For this review, take the finished solid that the model builds, in its own axes (mm). A direction names the side the tool comes from. Round coordinates to 2 decimals unless told otherwise and drop trailing zeros. Order: outer loops, then holes, each group sorted by start corner. A loop starts at its lowest first (then second) coordinate and runs counter-clockwise, first axis right, second up. Notation, with made-up numbers: (-6.75, 82.5) -> (41.25, 82.5) arc R13 ccw to (41.25, 92.5) -> close; hole circle Ø6 at (-21.75, -14). An arc over 180 degrees is marked (long way). Answer in a Markdown table with one row per item.
```python
from build123d import *

# Parameters (mm, degrees)
F1_DEPTH = 3.175


with BuildPart() as f1:
    # F0 (on Top) → F1 (new body)
    with BuildSketch(Plane.XY):
        with BuildLine():
            Line((-6.35, 51.198438), (-6.35, -101.6))
            Line((-6.35, -101.6), (-1.5875, -101.6))
            Line((-1.5875, -101.6), (-1.5875, 38.1))
            Line((-1.5875, 38.1), (1.5875, 38.1))
            Line((1.5875, 38.1), (1.5875, -101.6))
            Line((1.5875, -101.6), (6.35, -101.6))
            Line((6.35, -101.6), (6.35, 51.198438))
            ThreePointArc((6.35, 51.198438), (16.414418, 53.524987), (25.800126, 57.839361))
            Line((25.800126, 57.839361), (53.881537, 47.718463))
            Line((53.881537, 47.718463), (43.760639, 75.799874))
            ThreePointArc((43.760639, 75.799874), (46.93308, 82.159682), (49.186888, 88.9))
            Line((49.186888, 88.9), (76.2, 101.6))
            Line((76.2, 101.6), (49.186888, 114.3))
            ThreePointArc((49.186888, 114.3), (46.93308, 121.040318), (43.760639, 127.400126))
            Line((43.760639, 127.400126), (53.881537, 155.481537))
            Line((53.881537, 155.481537), (25.800126, 145.360639))
            ThreePointArc((25.800126, 145.360639), (19.440318, 148.53308), (12.7, 150.786888))
            Line((12.7, 150.786888), (0, 177.8))
            Line((0, 177.8), (-12.7, 150.786888))
            ThreePointArc((-12.7, 150.786888), (-19.440318, 148.53308), (-25.800126, 145.360639))
            Line((-25.800126, 145.360639), (-53.881537, 155.481537))
            Line((-53.881537, 155.481537), (-43.760639, 127.400126))
            ThreePointArc((-43.760639, 127.400126), (-46.93308, 121.040318), (-49.186888, 114.3))
            Line((-49.186888, 114.3), (-76.2, 101.6))
            Line((-76.2, 101.6), (-49.186888, 88.9))
            ThreePointArc((-49.186888, 88.9), (-46.93308, 82.159682), (-43.760639, 75.799874))
            Line((-43.760639, 75.799874), (-53.881537, 47.718463))
            Line((-53.881537, 47.718463), (-25.800126, 57.839361))
            ThreePointArc((-25.800126, 57.839361), (-16.414418, 53.524987), (-6.35, 51.198438))
        make_face()
    extrude(amount=F1_DEPTH)


solid = f1.part
```
Q1. Tool access review of faces 1 (the face through (62.5, 95.16, 1.57)), 2 (the face through (-39.64, 150.35, 1.57)), 3 (the face through (-62.5, 108.04, 1.57)), 4 (the face through (16.28, 53.48, 1.57)): name each direction out of +Z, -Z, +X, -X, +Y, -Y from which nothing blocks a thin tool from reaching the whole face with its end or side.
Answer key:
| item | result |
|---|---|
| face 1 | +Z, -Z, +X |
| face 2 | +Z, -Z, +Y |
| face 3 | +Z, -Z, -X |
| face 4 | +Z, -Z, -Y |
Q2. Take a section at C-C, the plane y = 54. Write out the cut boundary in (x, z) (3 decimals).
Answer key:
| item | result |
|---|---|
| outline | (-51.618, 0) -> (-36.453, 0) -> (-36.453, 3.175) -> (-51.618, 3.175) -> close; (-17.745, 0) -> (17.745, 0) -> (17.745, 3.175) -> (-17.745, 3.175) -> close; (36.453, 0) -> (51.618, 0) -> (51.618, 3.175) -> (36.453, 3.175) -> close |
Q3. The part is to be moulded in two halves that separate along Y. For faces 5 (the face through (46.895, 82.068, 1.565)), 6 (the face through (-40.037, 52.708, 1.565)), 7 (the face through (19.532, 148.495, 1.565)), say which applies: +Y half, -Y half, draft (parallel to the pull), parting line (faces both ways), or undercut.
Answer key:
| item | result |
|---|---|
| face 5 | undercut |
| face 6 | -Y half |
| face 7 | +Y half |
Q4. Take a section at D-D, the plane x = -62. Write out the cut boundary in (y, z) (3 decimals).
Answer key:
| item | result |
|---|---|
| outline | (94.924, 0) -> (108.276, 0) -> (108.276, 3.175) -> (94.924, 3.175) -> close |
Q5. To check wall thickness, follow probe 1 along X at (y, z) = (-60, 0.45); probe 2 along X at (y, z) = (43, 0.3); probe 3 along Y at (x, z) = (-38, 2.2). State the ranges of each line that lie inside material, in increasing order.
Answer key:
| item | result |
|---|---|
| probe 1 | x = -6.35 to -1.59, 1.59 to 6.35 |
| probe 2 | x = -6.35 to 6.35 |
| probe 3 | y = 53.44 to 149.76 |
Q6. Clearance check with flat-ended pins moving along their axes: pin 1 Ø1 at (y, z) = (-33, 2) entering from +X; pin 2 Ø1 at (x, z) = (41, 1) entering from +Y; pin 3 Ø1 at (y, z) = (-62.5, 1) entering from -X. State where each tip first meets the part, or that it passes through.
Answer key:
| item | result |
|---|---|
| pin 1 | stops at x = 6.35 |
| pin 2 | stops at y = 151.02 |
| pin 3 | stops at x = -6.35 |
